```python
from build123d import *

# Parameters (mm, degrees)
CROQUIS1_R                = 6.35
CROQUIS1_R_2              = 6.26
CROQUIS1_R_3              = 6.25
SALIENTE_EXTRUIR1_DEPTH   = 7.9375
CROQUIS2_W                = 150
CROQUIS2_H                = 104.1375
SALIENTE_EXTRUIR2_DEPTH   = 7.9375
CONVERTIR_S_LIDO1_START   = -75
CONVERTIR_S_LIDO1_DEPTH   = 150
CONVERTIR_S_LIDO1_2_DEPTH = 150


# Read off the part's stored shape, not the designer's step: Convertir-Sólido1
with BuildPart() as part:
    # Croquis1 → Saliente-Extruir1 (new body)
    with BuildSketch(Plane.XY):
        with BuildLine():
            Line((-75, 16), (-75, 0))
            Line((-75, 0), (75, 0))
            Line((75, 0), (75, 54))
            ThreePointArc((75, 54), (60.355339059, 89.355339059), (25, 104))
            Line((25, 104), (-200, 104))
            ThreePointArc((-200, 104), (-235.355339059, 89.355339059), (-250, 54))
            Line((-250, 54), (-250, 0))
            ThreePointArc((-250, 0), (0, -250), (250, 0))
            ThreePointArc((250, 0), (200, 50), (150, 0))
            ThreePointArc((150, 0), (0, -150), (-150, 0))
            Line((-150, 0), (-150, 16))
            Line((-150, 16), (-75, 16))
        make_face()
        with BuildLine():
            ThreePointArc((-49.374105038, 47.65), (-55.724105038, 54), (-49.374105038, 60.35))
            Line((-49.374105038, 60.35), (49.374105038, 60.35))
            ThreePointArc((49.374105038, 60.35), (55.724105038, 54), (49.374105038, 47.65))
            Line((49.374105038, 47.65), (-49.374105038, 47.65))
        make_face(mode=Mode.SUBTRACT)
        with Locations((193.014182094, -52.397762459)):
            Circle(CROQUIS1_R, mode=Mode.SUBTRACT)
        with Locations((200, 0)):
            Circle(CROQUIS1_R_2, mode=Mode.SUBTRACT)
        with Locations((-100, -173.205080757)):
            Circle(CROQUIS1_R_3, mode=Mode.SUBTRACT)
        with Locations((-52.397762459, -193.014182094)):
            Circle(CROQUIS1_R, mode=Mode.SUBTRACT)
        with Locations((-141.884884438, -140.956303754)):
            Circle(CROQUIS1_R, mode=Mode.SUBTRACT)
        with Locations((-173.205080757, -100)):
            Circle(CROQUIS1_R, mode=Mode.SUBTRACT)
        with Locations((0, -200)):
            Circle(CROQUIS1_R_3, mode=Mode.SUBTRACT)
        with Locations((51.129297656, -193.354066213)):
            Circle(CROQUIS1_R, mode=Mode.SUBTRACT)
        with Locations((100, -173.205080757)):
            Circle(CROQUIS1_R_3, mode=Mode.SUBTRACT)
        with Locations((140.956303754, -141.884884438)):
            Circle(CROQUIS1_R, mode=Mode.SUBTRACT)
        with Locations((173.205080757, -100)):
            Circle(CROQUIS1_R_3, mode=Mode.SUBTRACT)
        with Locations((-193.354066213, -51.129297656)):
            Circle(CROQUIS1_R, mode=Mode.SUBTRACT)
        with Locations((-200, 0)):
            Circle(CROQUIS1_R, mode=Mode.SUBTRACT)
        with Locations((-200, 54)):
            Circle(CROQUIS1_R, mode=Mode.SUBTRACT)
    extrude(amount=SALIENTE_EXTRUIR1_DEPTH)

    # Croquis2 → Saliente-Extruir2 (add)
    with BuildSketch(Plane.XZ):
        with Locations((0, -44.13125)):
            Rectangle(CROQUIS2_W, CROQUIS2_H)
        with BuildLine():
            Line((-50.16849794, -51.6), (50.16849794, -51.6))
            ThreePointArc((50.16849794, -51.6), (56.66849794, -58.1), (50.16849794, -64.6))
            Line((50.16849794, -64.6), (-50.16849794, -64.6))
            ThreePointArc((-50.16849794, -64.6), (-56.66849794, -58.1), (-50.16849794, -51.6))
        make_face(mode=Mode.SUBTRACT)
    extrude(amount=-SALIENTE_EXTRUIR2_DEPTH)

    # Convertir-Sólido1 outline → Convertir-Sólido1 (cut)
    with BuildSketch(Plane.YZ.offset(CONVERTIR_S_LIDO1_START)):
        with BuildLine():
            ThreePointArc((0, -4), (3.4964128, 4.4410872), (11.9375, 7.9375))
            Line((11.9375, 7.9375), (0, 7.9375))
            Line((0, 7.9375), (0, -4))
        make_face()
    extrude(amount=CONVERTIR_S_LIDO1_DEPTH, mode=Mode.SUBTRACT)

    # Convertir-S_lido1 2 outline → Convertir-S_lido1 2 (add)
    with BuildSketch(Plane.YZ.offset(CONVERTIR_S_LIDO1_START)):
        with BuildLine():
            Line((11.9375, 0), (7.9375, 0))
            Line((7.9375, 0), (7.9375, -4))
            ThreePointArc((7.9375, -4), (9.109072875, -1.171572875), (11.9375, 0))
        make_face()
    extrude(amount=CONVERTIR_S_LIDO1_2_DEPTH)


solid = part.part
```
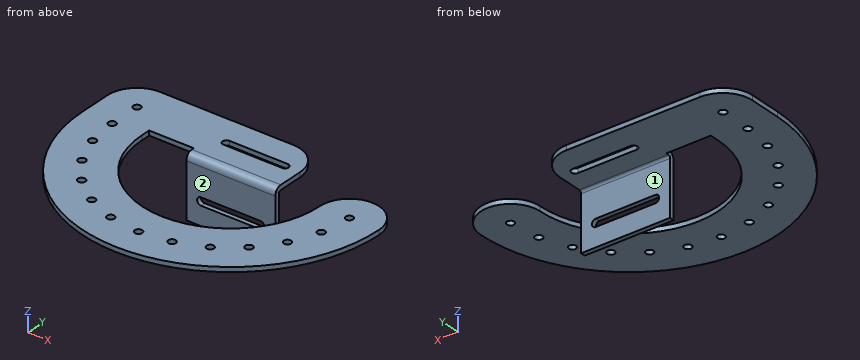
Could you check a few things on this model? Use its own coordinates, in mm. Face numbers are marked on the shaded views. A direction names the side the tool comes from. Coordinates: 2 decimals unless noted, no trailing zeros. Write each loop counter-clockwise with the first axis right and the second up, starting at its lowest first coordinate (ties: lowest second). Pieces come first, ordered by that corner, then holes. Notation, with made-up numbers: (37, -31.75) -> (47, -31.75) arc R21 cw to (47, -1.75) -> close; hole circle Ø11 at (22.25, 74.5). An arc over 180 degrees is marked (long way). Return JSON: item names as keys, results as strings.
(1) Imagine slicing it at A-A, the plane x = 0. Count the separate pieces of the cut face and the enclosed holes in it, then the cut area to 3 significant figures.
Numbers:
{"separate pieces": "5", "enclosed holes": "0", "area": "2,050 mm2"}
(2) Imagine slicing it at B-B, the plane y = -28.5. Please give me the cut outline in (x, z), then the cut area to 4 significant figures.
Numbers:
{"outline": "(-248.37, 0) -> (-147.27, 0) -> (-147.27, 7.94) -> (-248.37, 7.94) -> close; (147.27, 0) -> (248.37, 0) -> (248.37, 7.94) -> (147.27, 7.94) -> close", "area": "1,605 mm2"}
(3) Which directions (+Z, -Z, +X, -X, +Y, -Y) give clear straight access to the entire face, cutting with the end or side of a thin tool? Please do the marked faces 1 and 2.
Numbers:
{"face 1": "-Z, +X, -X, +Y", "face 2": "+Z, -Z, +X, -X, -Y"}
(4) I need wall thicknesses on L1, parallel to Z at x = 53.5, y = 75; L2, parallel to X at y = -220.5, z = 0.5. Which ranges of each line are inside material? Lowest first, please.
Numbers:
{"L1": "z = 0 to 7.94", "L2": "x = -117.81 to 117.81"}
(5) I'm going to push flat-ended pins straight in: pin 1 (16 mm diameter, centred on x = -100, y = -173.21, fed in from -Z); pin 2 (2.5 mm diameter, centred on y = 5.5, z = 4.5, fed in from +X); pin 3 (6 mm diameter, centred on x = 70, z = -74.5, fed in from +Y). Where does each tip first touch, or does it pass through?
Numbers:
{"pin 1": "stops at z = 0", "pin 2": "stops at x = 249.82", "pin 3": "stops at y = 7.94"}
(6) Imagine slicing it at C-C, the plane x = -100. Please give me the cut outline in (y, z), then the cut area to 3 significant figures.
Numbers:
{"outline": "(-229.13, 0) -> (-179.46, 0) -> (-179.46, 7.94) -> (-229.13, 7.94) -> close; (-166.96, 0) -> (-111.8, 0) -> (-111.8, 7.94) -> (-166.96, 7.94) -> close; (16, 0) -> (104, 0) -> (104, 7.94) -> (16, 7.94) -> close", "area": "1,530 mm2"}
(7) Imagine slicing it at D-D, the plane x = 100. Please give me the cut outline in (y, z).
Numbers:
{"outline": "(-229.13, 0) -> (-179.46, 0) -> (-179.46, 7.94) -> (-229.13, 7.94) -> close; (-166.96, 0) -> (-111.8, 0) -> (-111.8, 7.94) -> (-166.96, 7.94) -> close"}
